Geometry check sheet. Reference: the model listing, model coordinates, mm. Give positions to 0.01 mm unless a question says otherwise; leave off trailing zeros. Write each loop counter-clockwise with the first axis right and the second up, starting at its lowest first coordinate (ties: lowest second). Pieces come first, ordered by that corner, then holes.
(1) Cross-section at D-D (x = 56). Record the boundary of the cut face in (y, z).
(2) Cross-section at B-B (z = 82). Record the boundary of the cut face in (x, y), and give its area (3 significant figures).
(3) Cross-section at A-A (x = 131). Record the boundary of the cut face in (y, z), and give its area (3 significant figures).
(4) Cross-section at C-C (y = 0.85). Count the separate pieces of the cut face and the enclosed holes in it, and give its area (3 significant figures).
(5) Thickness scan on line 1 along X through (y, z) = (0.45, -15.5); line 2 along Z through (x, y) = (82, 0.6); line 3 along X through (y, z) = (0.8, 47). Record the ranges inside material, lowest first.
```python
from build123d import *

# Parameters (mm, degrees)
SKETCH1_W           = 1
SKETCH1_H           = 20
SKETCH1_W_2         = 20
SKETCH1_H_2         = 1
BOSS_EXTRUDE1_DEPTH = 1


with BuildPart() as part:
    # Sketch1 → Boss-Extrude1 (new body)
    with BuildSketch(Plane(origin=(0, 0, 0), x_dir=(1, 0, 0), z_dir=(0, 1, 0))):
        Polygon((0, 0), (100, 0), (100, -200), (150, -200), (150, 50), (0, 50), align=None)
        with Locations((5, 25)):
            Rectangle(SKETCH1_W, SKETCH1_H, mode=Mode.SUBTRACT)
        with Locations((30, 25)):
            Rectangle(SKETCH1_W, SKETCH1_H, mode=Mode.SUBTRACT)
        with Locations((95, 25)):
            Rectangle(SKETCH1_W, SKETCH1_H, mode=Mode.SUBTRACT)
        with Locations((125, -5)):
            Rectangle(SKETCH1_W_2, SKETCH1_H_2, mode=Mode.SUBTRACT)
        with Locations((125, -30)):
            Rectangle(SKETCH1_W_2, SKETCH1_H_2, mode=Mode.SUBTRACT)
        with Locations((125, -100)):
            Rectangle(SKETCH1_W_2, SKETCH1_H_2, mode=Mode.SUBTRACT)
        with Locations((125, -195)):
            Rectangle(SKETCH1_W_2, SKETCH1_H_2, mode=Mode.SUBTRACT)
        with Locations((125, -170)):
            Rectangle(SKETCH1_W_2, SKETCH1_H_2, mode=Mode.SUBTRACT)
        with Locations((125, 25)):
            Rectangle(SKETCH1_W_2, SKETCH1_H_2, mode=Mode.SUBTRACT)
        with Locations((70, 25)):
            Rectangle(SKETCH1_W, SKETCH1_H, mode=Mode.SUBTRACT)
    extrude(amount=BOSS_EXTRUDE1_DEPTH)


solid = part.part
```
Reply:
1. outline: (0, -50) - (1, -50) - (1, 0) - (0, 0) - close
2. outline: (100, 0) - (150, 0) - (150, 1) - (100, 1) - close
2. area: 50.0 mm2
3. outline: (0, -50) - (1, -50) - (1, -25.5) - (0, -25.5) - close; (0, -24.5) - (1, -24.5) - (1, 4.5) - (0, 4.5) - close; (0, 5.5) - (1, 5.5) - (1, 29.5) - (0, 29.5) - close; (0, 30.5) - (1, 30.5) - (1, 99.5) - (0, 99.5) - close; (0, 100.5) - (1, 100.5) - (1, 169.5) - (0, 169.5) - close; (0, 170.5) - (1, 170.5) - (1, 194.5) - (0, 194.5) - close; (0, 195.5) - (1, 195.5) - (1, 200) - (0, 200) - close
3. area: 244 mm2
4. separate pieces: 1
4. enclosed holes: 10
4. area: 17,300 mm2
5. line 1: x = 0 to 4.5, 5.5 to 29.5, 30.5 to 69.5, 70.5 to 94.5, 95.5 to 150
5. line 2: z = -50 to 0
5. line 3: x = 100 to 150
